from build123d import *

# Parameters (mm, degrees)
SKETCH1_R           = 1.77
BOSS_EXTRUDE1_DEPTH = 45


with BuildPart() as part:
    # Sketch1 → Boss-Extrude1 (new body)
    with BuildSketch(Plane.XY):
        Polygon((-8.38, 4.1), (-10, 4.1), (-10, 10), (-4.1, 10), (-4.1, 8.38), (-7.234487014, 8.38), (-2.954487014, 4.1), (2.954487014, 4.1), (7.234487014, 8.38), (4.1, 8.38), (4.1, 10), (10, 10), (10, 4.1), (8.38, 4.1), (8.38, 7.234487014), (4.1, 2.954487014), (4.1, -2.954487014), (8.38, -7.234487014), (8.38, -4.1), (10, -4.1), (10, -10), (4.1, -10), (4.1, -8.38), (7.234487014, -8.38), (2.954487014, -4.1), (-2.954487014, -4.1), (-7.234487014, -8.38), (-4.1, -8.38), (-4.1, -10), (-10, -10), (-10, -4.1), (-8.38, -4.1), (-8.38, -7.234487014), (-4.1, -2.954487014), (-4.1, 2.954487014), (-8.38, 7.234487014), align=None)
        with Locations(Location((0, 0, 0), (0, 0, 180))):
            Circle(SKETCH1_R, mode=Mode.SUBTRACT)
    extrude(amount=BOSS_EXTRUDE1_DEPTH)


solid = part.part
Part model, mm, in its own coordinate system. A direction names the side the tool comes from. Give positions to 0.01 mm unless a question says otherwise; leave off trailing zeros. Write each loop counter-clockwise with the first axis right and the second up, starting at its lowest first coordinate (ties: lowest second). Pieces come first, ordered by that corner, then holes.
1) Which spindle directions (+Z, -Z, +X, -X, +Y, -Y) get a long thin tool onto all of the face, cutting with end or side? Do faces 1 (the face through (4.1, 0, 22)), 2 (the face through (-5.124, 6.27, 22.185)), 3 (the face through (-4.1, 0, 22)). Say none if no direction does.
Resolved:
face 1: +Z, -Z, +X
face 2: +Z, -Z
face 3: +Z, -Z, -X
2) Two-plate mould, pull along Y, no slides. Class faces 4 (the face through (0, 4.1, 22)), 5 (the face through (-2, 0, 45)), 6 (the face through (8.38, 6, 22)): released by +Y, released by -Y, zero draft, split by the parting line, or undercut.
Resolved:
face 4: released by +Y
face 5: zero draft
face 6: undercut
3) Probe L1, parallel to Y at x = 0, z = 17.5; L2, parallel to Y at x = -5.75, z = 19.5; L3, parallel to Y at x = 6, z = 29. List the from-to ranges inside material, lowest first.
Resolved:
L1: y = -4.1 to -1.77, 1.77 to 4.1
L2: y = -10 to -8.38, -6.9 to -4.6, 4.6 to 6.9, 8.38 to 10
L3: y = -10 to -8.38, -7.15 to -4.85, 4.85 to 7.15, 8.38 to 10
4) Cut at A-A on y = 0. Write the cut outline in (x, z), then the cut area to 3 significant figures.
Resolved:
outline: (-4.1, 0) - (-1.77, 0) - (-1.77, 45) - (-4.1, 45) - close; (1.77, 0) - (4.1, 0) - (4.1, 45) - (1.77, 45) - close
area: 210 mm2
5) Pin check, flat tips, straight feed: pin 1 (3 mm diameter, centred on y = -2, z = 20.5, fed in from -X); pin 2 (3 mm diameter, centred on x = -0.5, z = 19.5, fed in from +Y); pin 3 (6.5 mm diameter, centred on y = -0.5, z = 17.5, fed in from -X). Stop position of each tip, or through.
Resolved:
pin 1: stops at x = -4.65
pin 2: stops at y = 4.1
pin 3: stops at x = -4.9
6) Cut at C-C on x = 6.5. Write the cut outline in (y, z).
Resolved:
outline: (-10, 0) - (-8.38, 0) - (-8.38, 45) - (-10, 45) - close; (-7.65, 0) - (-5.35, 0) - (-5.35, 45) - (-7.65, 45) - close; (5.35, 0) - (7.65, 0) - (7.65, 45) - (5.35, 45) - close; (8.38, 0) - (10, 0) - (10, 45) - (8.38, 45) - close
